```python
from build123d import *

# Parameters (mm, degrees)
F0_W          = 21.7
F0_H          = 21.7
F0_R          = 8.85
F1_DEPTH      = 10.85
F1_DEPTH_BACK = 10.85
F3_DEPTH      = 25


with BuildPart() as f1:
    # F0 (on Front) → F1 (new body, two sides)
    with BuildSketch(Plane.XZ) as f1_sk:
        Rectangle(F0_W, F0_H)
        Circle(F0_R, mode=Mode.SUBTRACT)
    extrude(amount=F1_DEPTH)
    extrude(f1_sk.sketch, amount=-F1_DEPTH_BACK)

    # F2 (on face) → F3 (cut)
    with BuildSketch(Plane.XY.offset(10.85)):
        with BuildLine():
            add(Edge.make_bspline(
                [(7.9357599601, -14.6792419255), (8.7533080621, -12.9220378395), (9.3575897376, -10.85)],
                knots=[0.8228915355, 0.8228915355, 0.8228915355, 1.0440868221, 1.0440868221, 1.0440868221], degree=2, weights=[1, 0.9938903122, 1]))
            Line((7.9357599601, -14.6792419255), (17.9156405647, -14.6792419255))
            Line((17.9156405647, -14.6792419255), (17.9156405647, 12.7848008303))
            Line((17.9156405647, 12.7848008303), (8.7213948385, 12.7848008303))
            add(Edge.make_bspline(
                [(9.3575897376, 10.85), (9.0655324995, 11.8514429913), (8.7213948385, 12.7848008303)],
                knots=[2.0975058315, 2.0975058315, 2.0975058315, 2.2047475395, 2.2047475395, 2.2047475395], degree=2, weights=[1, 0.9985627464, 1]))
            Line((9.3575897376, 10.85), (10.85, 10.85))
            Line((10.85, 10.85), (10.85, -10.85))
            Line((10.85, -10.85), (9.3575897376, -10.85))
        make_face()
        with BuildLine():
            Line((-17.9156405647, -14.6792419255), (-7.9357599601, -14.6792419255))
            add(Edge.make_bspline(
                [(-9.3575897376, -10.85), (-8.7533080621, -12.9220378395), (-7.9357599601, -14.6792419255)],
                knots=[5.2390984851, 5.2390984851, 5.2390984851, 5.4602937717, 5.4602937717, 5.4602937717], degree=2, weights=[1, 0.9938903122, 1]))
            Line((-9.3575897376, -10.85), (-10.85, -10.85))
            Line((-10.85, -10.85), (-10.85, 10.85))
            Line((-10.85, 10.85), (-9.3575897376, 10.85))
            add(Edge.make_bspline(
                [(-8.7213948385, 12.7848008303), (-9.0655324995, 11.8514429913), (-9.3575897376, 10.85)],
                knots=[4.0784377676, 4.0784377676, 4.0784377676, 4.1856794756, 4.1856794756, 4.1856794756], degree=2, weights=[1, 0.9985627464, 1]))
            Line((-8.7213948385, 12.7848008303), (-17.9156405647, 12.7848008303))
            Line((-17.9156405647, 12.7848008303), (-17.9156405647, -14.6792419255))
        make_face()
        with BuildLine():
            add(Edge.make_bspline(
                [(9.3575897376, -10.85), (12.5218447792, 0), (9.3575897376, 10.85)],
                knots=[1.0440868221, 1.0440868221, 1.0440868221, 2.0975058315, 2.0975058315, 2.0975058315], degree=2, weights=[1, 0.8644658516, 1]))
            Line((9.3575897376, -10.85), (10.85, -10.85))
            Line((10.85, -10.85), (10.85, 10.85))
            Line((10.85, 10.85), (9.3575897376, 10.85))
        make_face()
        with BuildLine():
            Line((-10.85, -10.85), (-9.3575897376, -10.85))
            add(Edge.make_bspline(
                [(-9.3575897376, 10.85), (-12.5218447792, 0), (-9.3575897376, -10.85)],
                knots=[4.1856794756, 4.1856794756, 4.1856794756, 5.2390984851, 5.2390984851, 5.2390984851], degree=2, weights=[1, 0.8644658516, 1]))
            Line((-9.3575897376, 10.85), (-10.85, 10.85))
            Line((-10.85, 10.85), (-10.85, -10.85))
        make_face()
    extrude(amount=-F3_DEPTH, mode=Mode.SUBTRACT)


solid = f1.part
```
The listing builds one solid part. Answer for the finished solid, in the listing's coordinates (mm). Round coordinates to 2 decimals unless told otherwise and drop trailing zeros. Write each loop counter-clockwise with the first axis right and the second up, starting at its lowest first coordinate (ties: lowest second). Pieces come first, ordered by that corner, then holes. Notation, with made-up numbers: (7.25, 87) -> (43.25, 87) arc R19 ccw to (43.25, 123) -> close; hole circle Ø8 at (9.25, 19.25). An arc over 180 degrees is marked (long way). Use CSV: the item, a comma, the result in double quotes. Start each with the question number.
(1) Each of these flat-tipped pins is pushed along its axis until it touches: pin 1 (5 mm diameter, centred on y = -4.5, z = 5, fed in from -X); pin 2 (2 mm diameter, centred on y = 3.5, z = 5, fed in from +X). Where does it stop, or does it pass through?
(2) Section A-A on x = 0 is taken. Give the vertices of the cut face in (y, z), then the cut area to 3 significant figures.
(3) The mould has two halves that part along Z. Classify faces 1 (the face through (0, 0, -10.85)), 2 (the face through (-6, -10.85, 7)), 3 (the face through (8.44, 0.15, 2.66)), 4 (the face through (0, 0, 10.85)): released by +Z, released by -Z, zero draft, split by the parting line, or undercut.
(4) Consider L1, parallel to Z at x = 0, y = 3.25; L2, parallel to X at y = 5, z = 2.75; L3, parallel to Z at x = -5.5, y = 5. Determine where each line is inside the solid, lowest interval first. Write a range as from..to.
(5) Section B-B on x = 4.75 is taken. Give the vertices of the cut face in (y, z), then the cut area to 3 significant figures.
A:
1,pin 1,"stops at x = -10.78"
1,pin 2,"stops at x = 10.75"
2,outline,"(-10.85, -10.85) -> (10.85, -10.85) -> (10.85, -8.85) -> (-10.85, -8.85) -> close; (-10.85, 8.85) -> (10.85, 8.85) -> (10.85, 10.85) -> (-10.85, 10.85) -> close"
2,area,"86.8 mm²"
3,face 1,"released by -Z"
3,face 2,"zero draft"
3,face 3,"undercut"
3,face 4,"released by +Z"
4,L1,"z = -10.85..-8.85, 8.85..10.85"
4,L2,"x = -10.53..-8.41, 8.41..10.53"
4,L3,"z = -10.85..-6.93, 6.93..10.85"
5,outline,"(-10.85, -10.85) -> (10.85, -10.85) -> (10.85, -7.47) -> (-10.85, -7.47) -> close; (-10.85, 7.47) -> (10.85, 7.47) -> (10.85, 10.85) -> (-10.85, 10.85) -> close"
5,area,"147 mm²"
